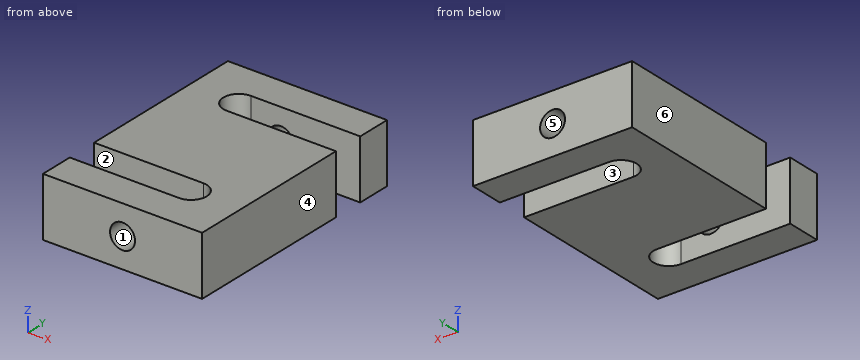
```python
from build123d import *

# Parameters (mm, degrees)
SKETCH_1_W          = 51
SKETCH_1_H          = 76
EXTRUDE_1_DEPTH     = 19
CUT_EXTRUDE_2_DEPTH = 50.550479312
SKETCH_2_R          = 4
CUT_EXTRUDE_1_DEPTH = 19


with BuildPart() as part:
    # 草图1 → 凸台-拉伸1 (new body)
    with BuildSketch(Plane.XY):
        Rectangle(SKETCH_1_W, SKETCH_1_H)
    extrude(amount=EXTRUDE_1_DEPTH)

    # 草图3 → 切除-拉伸2 (cut, through all)
    with BuildSketch(Plane(origin=(0, 0, 0), x_dir=(-1, 0, 0), z_dir=(0, 0, -1))):
        with BuildLine():
            Line((-25.5, 27), (9.5, 27))
            ThreePointArc((9.5, 27), (14.5, 22), (9.5, 17))
            Line((9.5, 17), (-25.5, 17))
            Line((-25.5, 17), (-25.5, 27))
        make_face()
        with BuildLine():
            Line((25.5, -27), (-9.5, -27))
            ThreePointArc((-9.5, -27), (-14.5, -22), (-9.5, -17))
            Line((-9.5, -17), (25.5, -17))
            Line((25.5, -17), (25.5, -27))
        make_face()
    extrude(amount=-CUT_EXTRUDE_2_DEPTH, mode=Mode.SUBTRACT)

    # 草图2 → 切除-拉伸1 (cut)
    with BuildSketch(Plane(origin=(0, 38, 0), x_dir=(1, 0, 0), z_dir=(0, 1, 0))):
        with Locations(Location((0, -9.5, 0), (0, 0, 270))):
            Circle(SKETCH_2_R)
    cut_extrude_1 = extrude(amount=-CUT_EXTRUDE_1_DEPTH, mode=Mode.SUBTRACT)

    # 镜向1: 切除-拉伸1 across plane
    add(cut_extrude_1.mirror(Plane.ZX), mode=Mode.SUBTRACT)


solid = part.part
```
Work out the finished part from the listing and answer in its coordinate system (mm). Face numbers are marked on the shaded views. A direction names the side the tool comes from. Give positions to 0.01 mm unless a question says otherwise; leave off trailing zeros. Loops run counter-clockwise (first coordinate to the right, second up) from the corner with the lowest first, then second, coordinate; pieces in that order, holes last. Notation, with made-up numbers: (-1, 11.25) -> (46, 11.25) arc R19 cw to (46, 48.25) -> close; hole circle Ø5 at (55.5, 73.25). An arc over 180 degrees is marked (long way). Write item = value, one per line. Start each with the question number.
(1) Which of the six approach directions +Z, -Z, +X, -X, +Y, -Y give full straight-line access (tool end or side, diameter ignored) to the marked faces 1, 2 and 3?
(2) Find section A-A on x = -18.5. Give the vertices of the cut face in (y, z), and give its area (3 significant figures).
(3) Given pin 1 Ø5 at (x, z) = (0, 9.5) entering from +Y, flat-ended and moving along its own axis, determine where the tip first touches the part or whether it passes through.
(4) Find section C-C on y = -31.5. Give the vertices of the cut face in (x, z).
(5) Find section B-B on z = 9.5. Give the vertices of the cut face in (x, y), and give its area (3 significant figures).
(6) Find section D-D on x = 0. Give the vertices of the cut face in (y, z), and give its area (3 significant figures).
(7) The mould has two halves that part along X. Classify the marked faces 4, 5 and 6: +X half, -X half, draft (parallel to the pull), parting line (faces both ways), or undercut.
(8) Find the intervals of material crossed by probe 1 along Y at (x, z) = (-2.5, 16.75); probe 2 along X at (y, z) = (-33.5, 9.5); probe 3 along Z at (x, y) = (0, -29), in increasing order. Write a range as from..to.
From the geometry:
q1.face_1 = -Y
q1.face_2 = +Z, -Z, -X
q1.face_3 = +Z, -Z, +X
q2.outline = (-38, 0) -> (-27, 0) -> (-27, 19) -> (-38, 19) -> close; (-17, 0) -> (38, 0) -> (38, 19) -> (-17, 19) -> close
q2.area = 1,250 mm^2
q3.pin_1 = 17
q4.outline = (-25.5, 0) -> (25.5, 0) -> (25.5, 19) -> (-25.5, 19) -> close; hole circle Ø8 at (0, 9.5)
q5.outline = (-25.5, -38) -> (-4, -38) -> (-4, -27) -> (-25.5, -27) -> close; (-25.5, -17) -> (9.5, -17) arc R5 cw to (9.5, -27) -> (4, -27) -> (4, -38) -> (25.5, -38) -> (25.5, 17) -> (-9.5, 17) arc R5 cw to (-9.5, 27) -> (-4, 27) -> (-4, 38) -> (-25.5, 38) -> close; (4, 27) -> (25.5, 27) -> (25.5, 38) -> (4, 38) -> close
q5.area = 2,920 mm^2
q6.outline = (-38, 0) -> (-27, 0) -> (-27, 5.5) -> (-38, 5.5) -> close; (-38, 13.5) -> (-27, 13.5) -> (-27, 19) -> (-38, 19) -> close; (-17, 0) -> (17, 0) -> (17, 19) -> (-17, 19) -> close; (27, 0) -> (38, 0) -> (38, 5.5) -> (27, 5.5) -> close; (27, 13.5) -> (38, 13.5) -> (38, 19) -> (27, 19) -> close
q6.area = 888 mm^2
q7.face_4 = +X half
q7.face_5 = undercut
q7.face_6 = -X half
q8.probe_1 = -38..-27, -17..17, 27..38
q8.probe_2 = -25.5..-4, 4..25.5
q8.probe_3 = 0..5.5, 13.5..19
